Model file for the job. Use its own axes, mm. A direction names the side the tool comes from. Give positions to 0.01 mm unless a question says otherwise; leave off trailing zeros. Loops run counter-clockwise (first coordinate to the right, second up) from the corner with the lowest first, then second, coordinate; pieces in that order, holes last. Notation, with made-up numbers: M 16,-4 L 71,-4 A32 cw 71,33 Z; hole C -36,46 d11. An arc over 180 degrees is marked long. Answer in a Markdown table with one row per item.
```python
from build123d import *

# Parameters (mm, degrees)
SKETCH2_W           = 160
SKETCH2_H           = 150
BOSS_EXTRUDE1_DEPTH = 60
CUT_EXTRUDE1_DEPTH  = 40
SKETCH4_R           = 3
CUT_EXTRUDE2_DEPTH  = 60
SKETCH5_W           = 13
SKETCH5_H           = 13
CUT_EXTRUDE3_DEPTH  = 50
SKETCH6_W           = 10
SKETCH6_H           = 53
CUT_EXTRUDE4_DEPTH  = 2
SKETCH7_W           = 35
SKETCH7_H           = 130
CUT_EXTRUDE5_DEPTH  = 40


with BuildPart() as part:
    # Sketch2 → Boss-Extrude1 (new body)
    with BuildSketch(Plane.XY):
        with Locations((-80, -75)):
            Rectangle(SKETCH2_W, SKETCH2_H)
    extrude(amount=BOSS_EXTRUDE1_DEPTH)

    # Sketch3 → Cut-Extrude1 (cut)
    with BuildSketch(Plane.XY.offset(60)):
        Polygon((-98.5, -10), (-23, -10), (-23, -140), (-157, -140), (-157, -100), (-98.5, -100), align=None)
    extrude(amount=-CUT_EXTRUDE1_DEPTH, mode=Mode.SUBTRACT)

    # Sketch4 → Cut-Extrude2 (cut)
    with BuildSketch(Plane.XY.offset(60)):
        with Locations((-103, -43)):
            Circle(SKETCH4_R)
        with Locations((-18, -43)):
            Circle(SKETCH4_R)
    extrude(amount=-CUT_EXTRUDE2_DEPTH, mode=Mode.SUBTRACT)

    # Sketch5 → Cut-Extrude3 (cut)
    with BuildSketch(Plane(origin=(0, 0, 0), x_dir=(0, 0, -1), z_dir=(1, 0, 0))):
        with Locations((-29.5, -121.5)):
            Rectangle(SKETCH5_W, SKETCH5_H)
    extrude(amount=-CUT_EXTRUDE3_DEPTH, mode=Mode.SUBTRACT)

    # Sketch6 → Cut-Extrude4 (cut)
    with BuildSketch(Plane.XY.offset(60)):
        with Locations((-103.5, -42.5)):
            Rectangle(SKETCH6_W, SKETCH6_H)
        with Locations((-18, -42.5)):
            Rectangle(SKETCH6_W, SKETCH6_H)
    extrude(amount=-CUT_EXTRUDE4_DEPTH, mode=Mode.SUBTRACT)

    # Sketch7 → Cut-Extrude5 (cut)
    with BuildSketch(Plane.XY.offset(60)):
        with Locations((-139.5, -75)):
            Rectangle(SKETCH7_W, SKETCH7_H)
    extrude(amount=-CUT_EXTRUDE5_DEPTH, mode=Mode.SUBTRACT)


solid = part.part
```
(1) Saw through at A-A, the plane x = -18. Give the cut face in (y, z), and give its area (3 significant figures).
Established:
| item | result |
|---|---|
| outline | M -150,0 L -46,0 L -46,58 L -69,58 L -69,60 L -150,60 Z; M -40,0 L 0,0 L 0,60 L -16,60 L -16,58 L -40,58 Z; hole M -128,23 L -115,23 L -115,36 L -128,36 Z |
| area | 8,380 mm2 |
(2) Flat gauge pins, fed straight in: P1, Ø6, axis at x = -35, z = 42, coming from the +Y side; P2, Ø5, axis at x = -103, y = -44.5, coming from the +Z side. Where does each tip first touch, or does it go through?
Established:
| item | result |
|---|---|
| P1 | stops at y = 0 |
| P2 | stops at z = 58 |
(3) Saw through at D-D, the plane x = -103. Give the cut face in (y, z), and give its area (3 significant figures).
Established:
| item | result |
|---|---|
| outline | M -150,0 L -46,0 L -46,58 L -69,58 L -69,60 L -100,60 L -100,20 L -140,20 L -140,60 L -150,60 Z; M -40,0 L 0,0 L 0,60 L -16,60 L -16,58 L -40,58 Z |
| area | 6,950 mm2 |
(4) Which spindle directions (+Z, -Z, +X, -X, +Y, -Y) get a long thin tool onto all of the face, cutting with end or side? Do faces 4 (the flat face through (-140, -10, 40)), 5 (the cylindrical face through (-20.21, -40.97, 29.41)), 6 (the flat face through (-11, -115, 30)). Say none if no direction does.
Established:
| item | result |
|---|---|
| face 4 | +Z |
| face 5 | +Z, -Z |
| face 6 | +X |
(5) Saw through at B-B, the plane y = -117.5. Give the cut face in (x, z).
Established:
| item | result |
|---|---|
| outline | M -160,0 L 0,0 L 0,23 L -23,23 L -23,20 L -157,20 L -157,60 L -160,60 Z; M -23,36 L 0,36 L 0,60 L -23,60 Z |
(6) Wall check: L1, parallel to X at y = -22.5, z = 54; L2, parallel to Y at x = -18, z = 35; L3, parallel to Y at x = -103, z = 43. Give the ranges that are in metal, low to high.
Established:
| item | result |
|---|---|
| L1 | x = -160 to -157, -122 to -98.5, -23 to 0 |
| L2 | y = -150 to -128, -115 to -46, -40 to 0 |
| L3 | y = -150 to -140, -100 to -46, -40 to 0 |
(7) Mould opens along Y. For faces 1 (the flat face through (-81, 0, 30)), 2 (the flat face through (-122, -56, 40)), 3 (the flat face through (-81, -74, 0)) say: pulls with the +Y half, pulls with the -Y half, needs draft (parallel to the pull), parting line crosses it, or undercut.
Established:
| item | result |
|---|---|
| face 1 | pulls with the +Y half |
| face 2 | undercut |
| face 3 | needs draft |
(8) Saw through at C-C, the plane z = 46. Give the cut face in (x, y), and give its area (3 significant figures).
Established:
| item | result |
|---|---|
| outline | M -160,-150 L 0,-150 L 0,0 L -160,0 Z; hole M -157,-140 L -23,-140 L -23,-10 L -98.5,-10 L -98.5,-100 L -122,-100 L -122,-10 L -157,-10 Z; hole C -103,-43 d6; hole C -18,-43 d6 |
| area | 8,640 mm2 |
